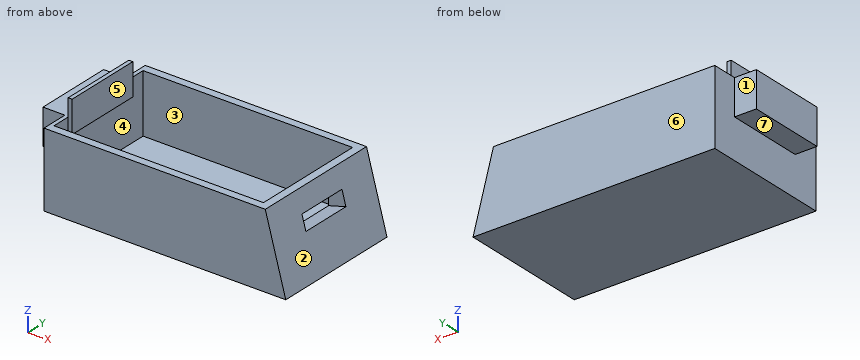
from build123d import *

# Parameters (mm, degrees)
F1_DEPTH = 21.209
F2_W     = 25.4
F2_H     = 11.43
F3_DEPTH = 7.0612
F4_W     = 16.764
F4_H     = 4.826
F5_DEPTH = 7.366
F6_W     = 67.564
F6_H     = 37.338
F7_DEPTH = 19.05
F8_W     = 25.4
F8_H     = 10.276243
F9_DEPTH = 1.27


with BuildPart() as f1:
    # F0 (on Front) → F1 (new body, symmetric)
    with BuildSketch(Plane.XZ):
        Polygon((-77.978, 0), (0, 0), (-6.604, 24.13), (-77.978, 24.13), align=None)
    extrude(amount=F1_DEPTH, both=True)

    # F2 (on face) → F3 (join)
    with BuildSketch(Plane(origin=(-77.978, 0, 0), x_dir=(0, -1, 0), z_dir=(-1, 0, 0))):
        with Locations((-0.254, 18.415)):
            Rectangle(F2_W, F2_H)
    extrude(amount=F3_DEPTH)

    # F4 (on face) → F5 (cut)
    with BuildSketch(Plane(origin=(0, 0, 0), x_dir=(0, 1, 0), z_dir=(0.964529, 0, 0.263976))):
        with Locations((0.254, 15.949588)):
            Rectangle(F4_W, F4_H)
    extrude(amount=-F5_DEPTH, mode=Mode.SUBTRACT)

    # F6 (on face) → F7 (cut)
    with BuildSketch(Plane.XY.offset(24.13)):
        with Locations((-42.926, 0)):
            Rectangle(F6_W, F6_H)
    extrude(amount=-F7_DEPTH, mode=Mode.SUBTRACT)

    # F8 (on face) → F9 (join)
    with BuildSketch(Plane.YZ.offset(-76.708)):
        with Locations((0, 24.579878)):
            Rectangle(F8_W, F8_H)
    extrude(amount=F9_DEPTH)


solid = f1.part
Input: part model. Units: mm. Frame: model coordinates. Face numbers are marked on the shaded views. A direction names the side the tool comes from. Give positions to 0.01 mm unless a question says otherwise; leave off trailing zeros. Loops run counter-clockwise (first coordinate to the right, second up) from the corner with the lowest first, then second, coordinate; pieces in that order, holes last. Notation, with made-up numbers: (17.5, 67) - (55.5, 67) arc R14 ccw to (55.5, 84) - close; hole circle Ø3 at (5, 77.5). An arc over 180 degrees is marked (long way). Use CSV: the item, a comma, the result in double quotes. Start each with the question number.
Item 1: Section A-A on y = 0. Return loops of the section in (x, z), then the cut area to 3 significant figures.
Item 2: Reachability of the marked faces 4, 5, 6 and 7 from +Z, -Z, +X, -X, +Y, -Y: full face, straight path, thin tool, end or side. Return the list, or none.
Item 3: Section B-B on x = -11. Return loops of the section in (y, z).
Item 4: Line query: line 1 (Y direction, x = -76.5, z = 19.5); line 2 (Z direction, x = -56, y = -1); line 3 (X direction, y = 12, z = 13). Output: solid intervals per line, ascending.
Item 5: Section C-C on z = 20.25. Return loops of the section in (x, y).
Item 6: Section D-D on y = -14. Return loops of the section in (x, z), then the cut area to 3 significant figures.
Item 7: Mould query, pull axis X, two halves, no side actions, for the marked faces 1, 2 and 3. Classes: pulls with the +X half, pulls with the -X half, needs draft (parallel to the pull), parting line crosses it, or undercut.
Item 8: Contact query for flat-ended pins moving along their axis: P1, Ø5.5, axis at y = -7.5, z = 10, coming from the +X side; P2, Ø3, axis at y = 4, z = 26.5, coming from the -X side; P3, Ø12.5, axis at x = -36.5, y = 4.5, coming from the +Z side; P4, Ø1.5, axis at x = -24, y = -0.5, coming from the -Z side. Output: stop coordinate, or through.
Ans:
1,outline,"(-85.04, 12.7) - (-77.98, 12.7) - (-77.98, 0) - (0, 0) - (-3.57, 13.06) - (-9.14, 11.53) - (-9.14, 5.08) - (-76.71, 5.08) - (-76.71, 19.44) - (-75.44, 19.44) - (-75.44, 29.72) - (-76.71, 29.72) - (-76.71, 24.13) - (-85.04, 24.13) - close; (-9.14, 16.54) - (-4.85, 17.71) - (-6.6, 24.13) - (-9.14, 24.13) - close"
1,area,"584 mm2"
2,face 4,"none"
2,face 5,"+Z"
2,face 6,"+Z, -Z, +X, -X, +Y"
2,face 7,"-Z, -X, +Y, -Y"
3,outline,"(-21.21, 0) - (21.21, 0) - (21.21, 24.13) - (18.67, 24.13) - (18.67, 5.08) - (-18.67, 5.08) - (-18.67, 24.13) - (-21.21, 24.13) - close"
4,line 1,"y = -21.21 to -18.67, -12.7 to 12.7, 18.67 to 21.21"
4,line 2,"z = 0 to 5.08"
4,line 3,"x = -85.04 to -76.71, -9.14 to -3.56"
5,outline,"(-85.04, -12.45) - (-77.98, -12.45) - (-77.98, -21.21) - (-5.54, -21.21) - (-5.54, 21.21) - (-77.98, 21.21) - (-77.98, 12.95) - (-85.04, 12.95) - close; hole (-76.71, -18.67) - (-9.14, -18.67) - (-9.14, 18.67) - (-76.71, 18.67) - (-76.71, 12.7) - (-75.44, 12.7) - (-75.44, -12.7) - (-76.71, -12.7) - close"
6,outline,"(-77.98, 0) - (0, 0) - (-6.6, 24.13) - (-9.14, 24.13) - (-9.14, 5.08) - (-76.71, 5.08) - (-76.71, 24.13) - (-77.98, 24.13) - close"
6,area,"515 mm2"
7,face 1,"needs draft"
7,face 2,"pulls with the +X half"
7,face 3,"undercut"
8,P1,"stops at x = -1.98"
8,P2,"stops at x = -76.71"
8,P3,"stops at z = 5.08"
8,P4,"stops at z = 0"
